Verification items for this drawing (mm, ordinates from the low corner). Give positions to 0.01 mm unless a question says otherwise; leave off trailing zeros. Order: outer loops, then holes, each group sorted by start corner. A loop starts at its lowest first (then second) coordinate and runs counter-clockwise, first axis right, second up.
(1) Gauge pin test, flat ends, axial feed: pin 1 (1.5 mm diameter, centred on x = 56.5, y = 17.5, fed in from +Z); pin 2 (4 mm diameter, centred on x = 40, y = 71, fed in from +Z); pin 3 (6 mm diameter, centred on x = 68.5, y = 39.5, fed in from +Z). Record the tip position at first contact, or that the pin passes through.
(2) Sectioned sample at D-D on y = 9.5. Record the cut outline in (x, z).
(3) Scan lines: L1, parallel to X at y = 36, z = 48; L2, parallel to Y at x = 66, z = 33.5; L3, parallel to X at y = 5.5, z = 24.5. Record each from-to range of solid material in increasing order.
(4) Sectioned sample at B-B on y = 55.5. Record the cut outline in (x, z), plus the area to 3 significant figures.
(5) Sectioned sample at A-A on x = 57. Record the cut outline in (y, z).
(6) Sectioned sample at C-C on z = 72. Record the cut outline in (x, y), plus the area to 3 significant figures.
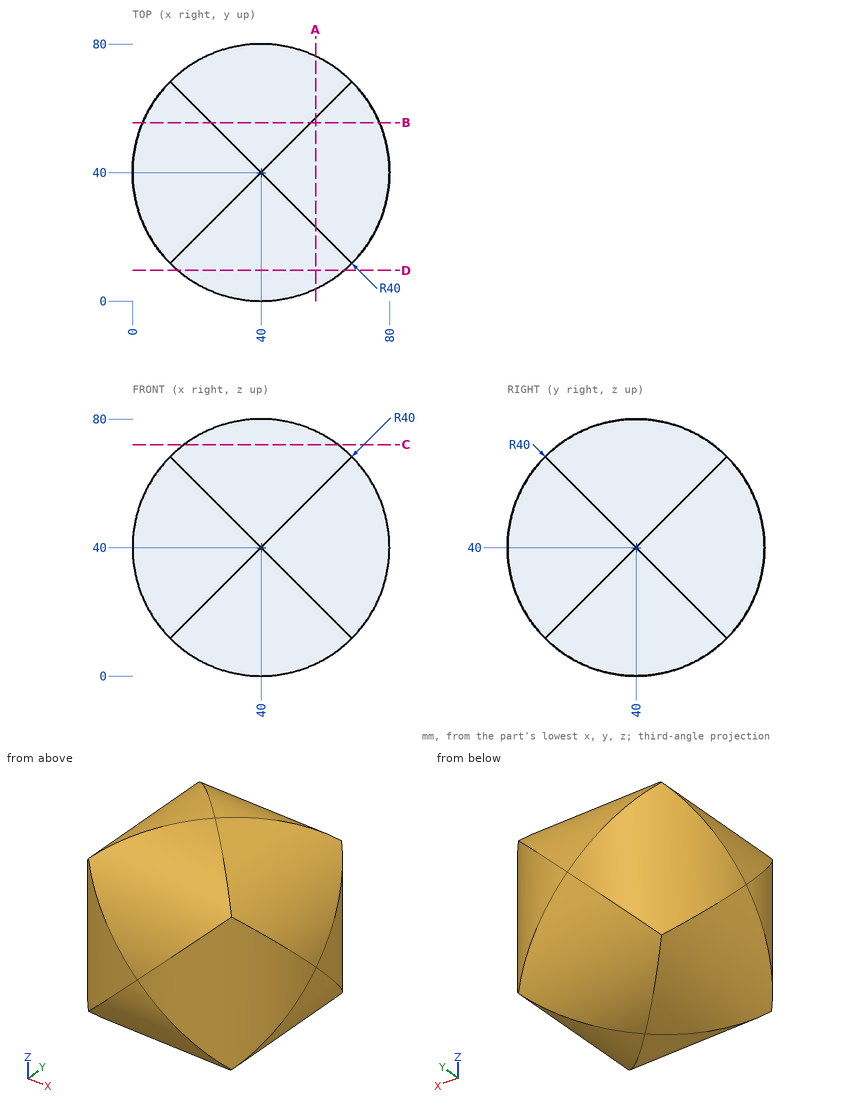
Ans:
1. pin 1: stops at z = 73.57
1. pin 2: stops at z = 67.55
1. pin 3: stops at z = 70.82
2. outline: (14.12, 14.12) - (65.88, 14.12) - (65.88, 65.88) - (14.12, 65.88) - close
3. L1: x = 0.81 to 79.19
3. L2: y = 9.6 to 70.4
3. L3: x = 19.76 to 60.24
4. outline: (3.13, 24.5) arc R40 ccw to (24.5, 3.13) - (55.5, 3.13) arc R40 ccw to (76.87, 24.5) - (76.87, 55.5) arc R40 ccw to (55.5, 76.87) - (24.5, 76.87) arc R40 ccw to (3.13, 55.5) - close
4. area: 4,770 mm2
5. outline: (3.79, 23) arc R40 ccw to (23, 3.79) - (57, 3.79) arc R40 ccw to (76.21, 23) - (76.21, 57) arc R40 ccw to (57, 76.21) - (23, 76.21) arc R40 ccw to (3.79, 57) - close
6. outline: (16, 16) - (64, 16) - (64, 64) - (16, 64) - close
6. area: 2,300 mm2
